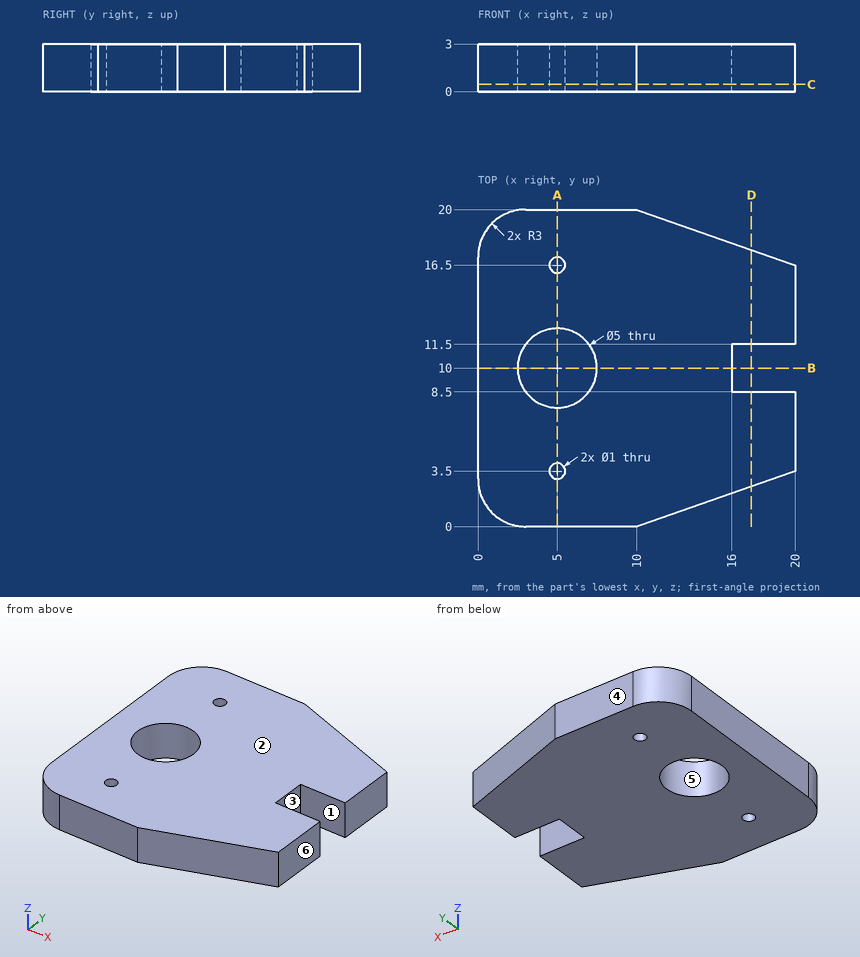
Geometry: see drawing. Coordinates: mm, zero at the bounding-box minimum. A direction names the side the tool comes from. Coordinates: 2 decimals unless noted, no trailing zeros. Write each loop counter-clockwise with the first axis right and the second up, starting at its lowest first coordinate (ties: lowest second). Pieces come first, ordered by that corner, then holes. Notation, with made-up numbers: (-0.5, 13.5) - (45.5, 13.5) arc R21 cw to (45.5, 42.5) - close; hole circle Ø9 at (9.5, 47.25). An arc over 180 degrees is marked (long way). Put each result on its own line as item: value. Start each with the question number.
1) Reachability of the marked faces 1 and 2 from +Z, -Z, +X, -X, +Y, -Y: full face, straight path, thin tool, end or side. Return the list, or none.
2) Cut plane D-D (x = 17.25). Return the cut outline in (y, z).
3) Cut plane C-C (z = 0.45). Return the cut outline in (x, y).
4) Ray query, L1, parallel to Y at x = 5, z = 0.6; L2, parallel to X at y = 12, z = 2.25; L3, parallel to Y at x = 2, z = 2.3. Return the intervals inside material, ascending.
5) Cut plane A-A (x = 5). Return the cut outline in (y, z).
6) Cut plane B-B (y = 10). Return the cut outline in (x, z), plus the area to 3 significant figures.
7) Mould query, pull axis Y, two halves, no side actions, for the marked faces 3, 4, 5 and 6. Classes: pulls with the +Y half, pulls with the -Y half, needs draft (parallel to the pull), parting line crosses it, or undercut.
Resolved:
1. face 1: +Z, -Z, +X
1. face 2: +Z, +X, -X, +Y, -Y
2. outline: (2.54, 0) - (8.5, 0) - (8.5, 3) - (2.54, 3) - close; (11.5, 0) - (17.46, 0) - (17.46, 3) - (11.5, 3) - close
3. outline: (0, 3) arc R3 ccw to (3, 0) - (10, 0) - (20, 3.5) - (20, 8.5) - (16, 8.5) - (16, 11.5) - (20, 11.5) - (20, 16.5) - (10, 20) - (3, 20) arc R3 ccw to (0, 17) - close; hole circle Ø5 at (5, 10); hole circle Ø1 at (5, 3.5); hole circle Ø1 at (5, 16.5)
4. L1: y = 0 to 3, 4 to 7.5, 12.5 to 16, 17 to 20
4. L2: x = 0 to 3.5, 6.5 to 20
4. L3: y = 0.17 to 19.83
5. outline: (0, 0) - (3, 0) - (3, 3) - (0, 3) - close; (4, 0) - (7.5, 0) - (7.5, 3) - (4, 3) - close; (12.5, 0) - (16, 0) - (16, 3) - (12.5, 3) - close; (17, 0) - (20, 0) - (20, 3) - (17, 3) - close
6. outline: (0, 0) - (2.5, 0) - (2.5, 3) - (0, 3) - close; (7.5, 0) - (16, 0) - (16, 3) - (7.5, 3) - close
6. area: 33.0 mm2
7. face 3: undercut
7. face 4: pulls with the +Y half
7. face 5: undercut
7. face 6: needs draft
